Read the model definition and answer for the solid it produces. Units are mm, in the model's axes. Face numbers are marked on the shaded views. Round coordinates to 2 decimals unless told otherwise and drop trailing zeros. Order: outer loops, then holes, each group sorted by start corner. A loop starts at its lowest first (then second) coordinate and runs counter-clockwise, first axis right, second up. Notation, with made-up numbers: (-39.5, 87.5) - (0.5, 87.5) arc R24 cw to (0.5, 113.5) - close; hole circle Ø1 at (23.5, 76.5). An arc over 180 degrees is marked (long way). One line per question, with ' | ' between items. Start each with the question number.
1) The part is cut by section C-C, the plane x = 4. Give the vertices of the cut face in (y, z), plus the area to 3 significant figures.
2) The part is cut by section D-D, the plane z = 4.5. Give the vertices of the cut face in (x, y), plus the area to 3 significant figures.
3) A flat-ended cylindrical pin translates along its axis: pin 1 (2 mm diameter, centred on x = 37.61, y = -29.93, fed in from -Z). Find the tip coordinate at first contact, or state that the pin passes through.
4) The part is cut by section B-B, the plane y = -32.5. Give the vertices of the cut face in (x, z), plus the area to 3 significant figures.
5) Straight lines are drawn through the part: line 1 (X direction, y = -31, z = 9); line 2 (Y direction, x = 16.5, z = 7); line 3 (Y direction, x = 38, z = 8). For each, find the intervals that lie inside material, in ascending order. Write a range as from..to.
6) The mould has two halves that part along Y. Classify the marked faces 1, 2, 3 and 4: pulls with the +Y half, pulls with the -Y half, needs draft (parallel to the pull), parting line crosses it, or undercut.
7) The part is cut by section A-A, the plane z = 16. Count the separate pieces of the cut face and the enclosed holes in it, plus the area to 3 significant figures.
from build123d import *

# Parameters (mm, degrees)
SKETCH1_W           = 48.9
SKETCH1_H           = 36.3
BOSS_EXTRUDE1_DEPTH = 26
CUT_EXTRUDE1_DEPTH  = 24.5
SKETCH4_W           = 2.15
SKETCH4_H           = 2.35
BOSS_EXTRUDE3_DEPTH = 24.5
SKETCH5_W           = 26.82
SKETCH5_H           = 2.95
BOSS_EXTRUDE4_DEPTH = 16.12
SKETCH6_W           = 4.57
SKETCH6_H           = 0.74
SKETCH6_W_2         = 8
CUT_EXTRUDE2_DEPTH  = 16.12
SKETCH7_W           = 38.3
SKETCH7_H           = 36.3
BOSS_EXTRUDE5_DEPTH = 48.9
SKETCH8_R           = 0.9
CUT_EXTRUDE3_DEPTH  = 11.45
SKETCH9_R           = 0.8
CUT_EXTRUDE4_DEPTH  = 71.719887585


with BuildPart() as part:
    # Sketch1 → Boss-Extrude1 (new body)
    with BuildSketch(Plane.XY):
        with Locations((24.45, -18.15)):
            Rectangle(SKETCH1_W, SKETCH1_H)
    extrude(amount=BOSS_EXTRUDE1_DEPTH)

    # Sketch3 → Cut-Extrude1 (cut)
    with BuildSketch(Plane(origin=(0, 0, 0), x_dir=(-1, 0, 0), z_dir=(0, 0, -1))):
        Polygon((-24.45, -1.98), (-46.92, -1.98), (-46.92, -34.32), (-1.98, -34.32), (-1.98, -1.98), align=None)
    extrude(amount=-CUT_EXTRUDE1_DEPTH, mode=Mode.SUBTRACT)

    # Sketch4 → Boss-Extrude3 (add)
    with BuildSketch(Plane(origin=(0, 0, 24.5), x_dir=(-1, 0, 0), z_dir=(0, 0, -1))):
        with Locations((-38.585, -3.155)):
            Rectangle(SKETCH4_W, SKETCH4_H)
        with Locations((-29.485, -3.155)):
            Rectangle(SKETCH4_W, SKETCH4_H)
        with Locations((-20.385, -3.155)):
            Rectangle(SKETCH4_W, SKETCH4_H)
        with Locations((-11.285, -3.155)):
            Rectangle(SKETCH4_W, SKETCH4_H)
    extrude(amount=BOSS_EXTRUDE3_DEPTH)

    # Sketch5 → Boss-Extrude4 (add)
    with BuildSketch(Plane(origin=(0, 0, 24.5), x_dir=(-1, 0, 0), z_dir=(0, 0, -1))):
        with Locations((-24.45, -18.845)):
            Rectangle(SKETCH5_W, SKETCH5_H)
    extrude(amount=BOSS_EXTRUDE4_DEPTH)

    # Sketch6 → Cut-Extrude2 (cut)
    with BuildSketch(Plane(origin=(0, 0, 8.38), x_dir=(-1, 0, 0), z_dir=(0, 0, -1))):
        with Locations((-33.205, -19.95)):
            Rectangle(SKETCH6_W, SKETCH6_H)
        with Locations((-24.55, -19.95)):
            Rectangle(SKETCH6_W_2, SKETCH6_H)
        with Locations((-15.695, -19.95)):
            Rectangle(SKETCH6_W, SKETCH6_H)
        with Locations((-15.695, -17.74)):
            Rectangle(SKETCH6_W, SKETCH6_H)
        with Locations((-24.55, -17.74)):
            Rectangle(SKETCH6_W_2, SKETCH6_H)
        with Locations((-33.205, -17.74)):
            Rectangle(SKETCH6_W, SKETCH6_H)
    extrude(amount=-CUT_EXTRUDE2_DEPTH, mode=Mode.SUBTRACT)

    # Sketch7 → Boss-Extrude5 (add)
    with BuildSketch(Plane(origin=(48.9, 0, 0), x_dir=(0, 0, -1), z_dir=(1, 0, 0))):
        with Locations((-45.15, -18.15)):
            Rectangle(SKETCH7_W, SKETCH7_H)
    extrude(amount=-BOSS_EXTRUDE5_DEPTH)

    # Sketch8 → Cut-Extrude3 (cut)
    with BuildSketch(Plane(origin=(0, 0, 24.5), x_dir=(-1, 0, 0), z_dir=(0, 0, -1))):
        with Locations((-37.61143404, -29.928818747)):
            Circle(SKETCH8_R)
        with Locations((-15.010991749, -29.088008467)):
            Circle(SKETCH8_R)
    extrude(amount=-CUT_EXTRUDE3_DEPTH, mode=Mode.SUBTRACT)

    # Sketch9 → Cut-Extrude4 (cut, through all)
    with BuildSketch(Plane(origin=(0, 0, 35.95), x_dir=(-1, 0, 0), z_dir=(0, 0, -1))):
        with Locations((-37.61143404, -29.928818747)):
            Circle(SKETCH9_R)
        with Locations((-15.010991749, -29.088008467)):
            Circle(SKETCH9_R)
    extrude(amount=-CUT_EXTRUDE4_DEPTH, mode=Mode.SUBTRACT)


solid = part.part
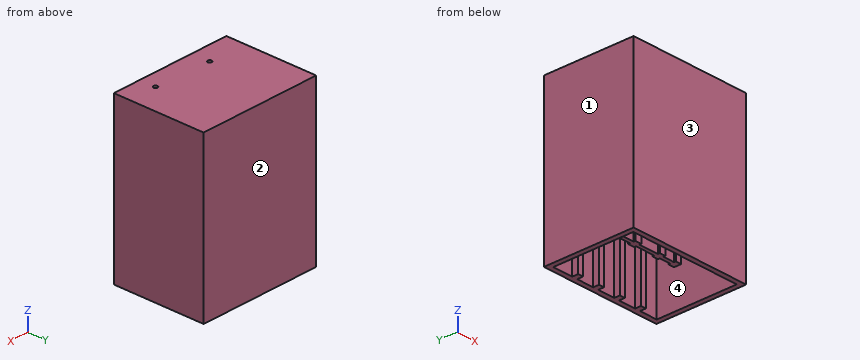
Values:
1) outline: (-36.3, 0) - (-34.32, 0) - (-34.32, 24.5) - (-1.98, 24.5) - (-1.98, 0) - (0, 0) - (0, 64.3) - (-36.3, 64.3) - close | area: 1,540 mm^2
2) outline: (0, -36.3) - (48.9, -36.3) - (48.9, 0) - (0, 0) - close; hole (1.98, -34.32) - (46.92, -34.32) - (46.92, -1.98) - (39.66, -1.98) - (39.66, -4.33) - (37.51, -4.33) - (37.51, -1.98) - (30.56, -1.98) - (30.56, -4.33) - (28.41, -4.33) - (28.41, -1.98) - (21.46, -1.98) - (21.46, -4.33) - (19.31, -4.33) - (19.31, -1.98) - (12.36, -1.98) - (12.36, -4.33) - (10.21, -4.33) - (10.21, -1.98) - (1.98, -1.98) - close | area: 342 mm^2
3) pin 1: stops at z = 24.5
4) outline: (0, 0) - (1.98, 0) - (1.98, 24.5) - (46.92, 24.5) - (46.92, 0) - (48.9, 0) - (48.9, 64.3) - (0, 64.3) - close | area: 2,040 mm^2
5) line 1: x = 0..1.98, 46.92..48.9 | line 2: y = -36.3..-34.32, -1.98..0 | line 3: y = -36.3..-34.32, -4.33..0
6) face 1: needs draft | face 2: pulls with the +Y half | face 3: pulls with the -Y half | face 4: undercut
7) separate pieces: 2 | enclosed holes: 1 | area: 396 mm^2
